Model file for the job. Use its own axes, mm. Face numbers are marked on the shaded views. A direction names the side the tool comes from. Give positions to 0.01 mm unless a question says otherwise; leave off trailing zeros. Write each loop counter-clockwise with the first axis right and the second up, starting at its lowest first coordinate (ties: lowest second). Pieces come first, ordered by that corner, then holes. Notation, with made-up numbers: (3.25, 88.5) - (47.25, 88.5) arc R20 ccw to (47.25, 109.5) - close; hole circle Ø9 at (86, -37.75). An arc over 180 degrees is marked (long way). One line per item, written item: value. Start each with the question number.
(1) Cut at A-A, the plane y = 4.25. List the corners of the cut face in (x, z).
(2) 3-axis set-ups, long thin cutter, end or side, ignore diameter. For the marked faces 4, 5, 6, 7 and 8: which of +Z, -Z, +X, -X, +Y, -Y reach the whole face in a straight line?
(3) Drop flat-ended pins along their axis: P1, Ø1.2, axis at y = 2, z = 2.5, coming from the +X side; P2, Ø1, axis at x = -5, y = 3, coming from the -Z side; P3, Ø3.5, axis at x = -2, z = -1, coming from the +Y side; P4, Ø3, axis at x = 2, z = 0.5, coming from the -Y side. Give the stop position or say it passes through.
(4) Mould opens along X. For the marked faces 1, 2 and 3 say: pulls with the +X half, pulls with the -X half, needs draft (parallel to the pull), parting line crosses it, or undercut.
(5) Cut at D-D, the plane x = 5.25. List the corners of the cut face in (y, z), and give its area (3 significant figures).
(6) Cut at C-C, the plane z = -1.5. List the corners of the cut face in (x, y).
(7) Probe L1, parallel to Y at x = -6.25, z = 0.75; L2, parallel to X at y = 5.25, z = 2.25; L3, parallel to Z at x = -3.75, y = 3.75. List the from-to ranges inside material, lowest first.
(8) Cut at B-B, the plane y = 2.5. List the corners of the cut face in (x, z).
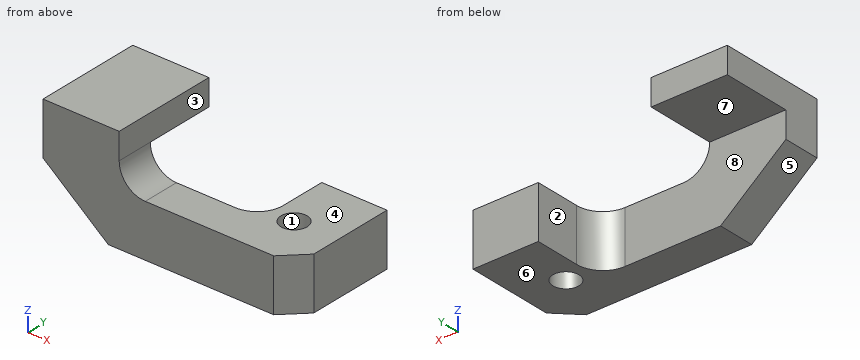
from build123d import *

# Parameters (mm, degrees)
SKETCH1_W           = 14.732
SKETCH1_H           = 6.096
BOSS_EXTRUDE1_DEPTH = 6.35
CUT_EXTRUDE2_DEPTH  = 7.35
SKETCH3_W           = 10.922
SKETCH3_H           = 6.096
CUT_EXTRUDE1_DEPTH  = 2.667
CUT_EXTRUDE3_DEPTH  = 4.683
SKETCH9_W           = 4.445
SKETCH9_H           = 1.524
BOSS_EXTRUDE2_DEPTH = 2.54
CUT_EXTRUDE4_DEPTH  = 7.096
CUT_EXTRUDE5_DEPTH  = 4.191
SKETCH15_W          = 0.048393345
SKETCH15_H          = 1.524
CUT_EXTRUDE10_DEPTH = 2.905
SKETCH13_W          = 4.445
SKETCH13_H          = 1.524
CUT_EXTRUDE11_DEPTH = 4.572
SKETCH16_R          = 0.762
CUT_EXTRUDE12_DEPTH = 4.572


with BuildPart() as part:
    # Sketch1 → Boss-Extrude1 (new body)
    with BuildSketch(Plane(origin=(0, 0, 0), x_dir=(1, 0, 0), z_dir=(0, 1, 0))):
        Rectangle(SKETCH1_W, SKETCH1_H)
    extrude(amount=BOSS_EXTRUDE1_DEPTH)

    # Sketch4 → Cut-Extrude2 (cut, through all)
    with BuildSketch(Plane(origin=(0, 6.35, 0), x_dir=(1, 0, 0), z_dir=(0, 1, 0))):
        with BuildLine():
            Line((7.366, 0), (-1.397, 0))
            ThreePointArc((-1.397, 0), (-0.319369265, -0.446369265), (0.127, -1.524))
            ThreePointArc((0.127, -1.524), (-0.319369265, -2.601630735), (-1.397, -3.048))
            Line((-1.397, -3.048), (7.366, -3.048))
            Line((7.366, -3.048), (7.366, 0))
        make_face()
        with BuildLine():
            ThreePointArc((0.127, -1.524), (-0.319369265, -0.446369265), (-1.397, 0))
            Line((-1.397, 0), (-1.397, -3.048))
            ThreePointArc((-1.397, -3.048), (-0.319369265, -2.601630735), (0.127, -1.524))
        make_face()
        with BuildLine():
            Line((-1.397, -3.048), (-1.397, 0))
            ThreePointArc((-1.397, 0), (-2.474630735, -0.446369265), (-2.921, -1.524))
            ThreePointArc((-2.921, -1.524), (-2.474630735, -2.601630735), (-1.397, -3.048))
        make_face()
        with BuildLine():
            ThreePointArc((-1.397, -3.048), (-2.474630735, -2.601630735), (-2.921, -1.524))
            Line((-2.921, -1.524), (-2.921, -3.048))
            Line((-2.921, -3.048), (-1.397, -3.048))
        make_face()
    extrude(amount=-CUT_EXTRUDE2_DEPTH, mode=Mode.SUBTRACT)

    # Sketch3 → Cut-Extrude1 (cut)
    with BuildSketch(Plane(origin=(0, 6.35, 0), x_dir=(1, 0, 0), z_dir=(0, 1, 0))):
        with Locations((-1.905, 0)):
            Rectangle(SKETCH3_W, SKETCH3_H)
    extrude(amount=-CUT_EXTRUDE1_DEPTH, mode=Mode.SUBTRACT)

    # Sketch8 → Cut-Extrude3 (cut, through all)
    with BuildSketch(Plane(origin=(0, 3.683, 0), x_dir=(1, 0, 0), z_dir=(0, 1, 0))):
        Polygon((-7.366, 0), (-3.556, 3.048), (-7.366, 3.048), align=None)
    extrude(amount=-CUT_EXTRUDE3_DEPTH, mode=Mode.SUBTRACT)

    # Sketch9 → Boss-Extrude2 (add)
    with BuildSketch(Plane(origin=(0, 3.683, 0), x_dir=(1, 0, 0), z_dir=(0, 1, 0))):
        with Locations((-5.1435, -2.286)):
            Rectangle(SKETCH9_W, SKETCH9_H)
    extrude(amount=BOSS_EXTRUDE2_DEPTH)

    # Sketch10 → Cut-Extrude4 (cut, through all)
    with BuildSketch(Plane(origin=(0, 0, -3.048), x_dir=(-1, 0, 0), z_dir=(0, 0, -1))):
        Polygon((-7.366, 1.27), (-6.096, 0), (-7.366, 0), align=None)
    extrude(amount=-CUT_EXTRUDE4_DEPTH, mode=Mode.SUBTRACT)

    # Sketch12 → Cut-Extrude5 (cut)
    with BuildSketch(Plane(origin=(0, 0, -3.048), x_dir=(-1, 0, 0), z_dir=(0, 0, -1))):
        with BuildLine():
            ThreePointArc((-3.556, 3.683), (-3.109630735, 2.605369265), (-2.032, 2.159))
            Line((-2.032, 2.159), (2.921, 2.159))
            Line((2.921, 2.159), (2.921, 3.683))
            Line((2.921, 3.683), (-3.556, 3.683))
        make_face()
    extrude(amount=-CUT_EXTRUDE5_DEPTH, mode=Mode.SUBTRACT)

    # Sketch15 → Cut-Extrude10 (cut, through all)
    with BuildSketch(Plane(origin=(0, 0, 1.143), x_dir=(-1, 0, 0), z_dir=(0, 0, -1))):
        with Locations((2.896803328, 2.921)):
            Rectangle(SKETCH15_W, SKETCH15_H)
    extrude(amount=-CUT_EXTRUDE10_DEPTH, mode=Mode.SUBTRACT)

    # Sketch13 → Cut-Extrude11 (cut)
    with BuildSketch(Plane(origin=(0, 0, -3.048), x_dir=(-1, 0, 0), z_dir=(0, 0, -1))):
        with Locations((5.1435, 2.921)):
            Rectangle(SKETCH13_W, SKETCH13_H)
    extrude(amount=-CUT_EXTRUDE11_DEPTH, mode=Mode.SUBTRACT)

    # Sketch16 → Cut-Extrude12 (cut)
    with BuildSketch(Plane(origin=(0, 0, -3.048), x_dir=(-1, 0, 0), z_dir=(0, 0, -1))):
        with Locations((-4.826, 2.921)):
            Circle(SKETCH16_R)
    extrude(amount=-CUT_EXTRUDE12_DEPTH, mode=Mode.SUBTRACT)


solid = part.part
Answers follow:
1. outline: (-7.37, 1.52) - (-2.92, 1.52) - (-2.92, 3.05) - (-7.37, 3.05) - close; (3.56, -3.05) - (7.37, -3.05) - (7.37, 0) - (3.56, 0) - close
2. face 4: +Z, +X, +Y, -Y
2. face 5: -Z, -X, +Y, -Y
2. face 6: -Z, +X, -X, +Y, -Y
2. face 7: -Z, +X, -X, +Y
2. face 8: -Z, -X, +Y
3. P1: stops at x = -2.92
3. P2: stops at z = 1.52
3. P3: stops at y = 2.16
3. P4: stops at y = 0
4. face 1: undercut
4. face 2: pulls with the -X half
4. face 3: pulls with the +X half
5. outline: (0, -3.05) - (2.29, -3.05) - (2.29, 0) - (0, 0) - close; (3.55, -3.05) - (6.35, -3.05) - (6.35, 0) - (3.55, 0) - close
5. area: 15.5 mm²
6. outline: (-5.49, 0) - (6.1, 0) - (7.37, 1.27) - (7.37, 6.35) - (3.56, 6.35) - (3.56, 3.68) arc R1.52 cw to (2.03, 2.16) - (-5.49, 2.16) - close; hole circle Ø1.52 at (4.83, 2.92)
7. L1: y = 0 to 2.16
7. L2: x = -7.37 to -2.92
7. L3: z = 1.52 to 3.05
8. outline: (-7.37, 1.52) - (-2.92, 1.52) - (-2.92, 3.05) - (-7.37, 3.05) - close; (2.99, -3.05) - (4.19, -3.05) - (4.19, 0) - (2.99, 0) - close; (5.46, -3.05) - (7.37, -3.05) - (7.37, 0) - (5.46, 0) - close
